```python
from build123d import *

# Parameters (mm, degrees)
SKETCH1_W                = 90
SKETCH1_H                = 29
SKETCH1_W_2              = 86
SKETCH1_H_2              = 25
BOSS_EXTRUDE1_DEPTH      = 12
SKETCH1_2_W              = 90
SKETCH1_2_H              = 29
SKETCH1_2_W_2            = 86
SKETCH1_2_H_2            = 25
BOSS_EXTRUDE2_DEPTH      = 2
SKETCH2_R                = 1
BOSS_EXTRUDE3_DEPTH      = 2.65
SKETCH3_R                = 1.75
BOSS_EXTRUDE4_DEPTH      = 1
CHAMFER1_SIZE            = 1
CUT_EXTRUDE1_REACH       = 55.833
SKETCH4_W                = 13
SKETCH4_H                = 10
CUT_EXTRUDE2_REACH       = 56.863
SKETCH5_W                = 24
SKETCH5_H                = 3
CHAMFER2_SIZE            = 1
CHAMFER2_OF_MIRROR2_SIZE = 1


with BuildPart() as part:
    # Sketch1 → Boss-Extrude1 (new body)
    with BuildSketch(Plane(origin=(0, 0, 0), x_dir=(1, 0, 0), z_dir=(0, 1, 0))):
        Rectangle(SKETCH1_W, SKETCH1_H)
        Rectangle(SKETCH1_W_2, SKETCH1_H_2, mode=Mode.SUBTRACT)
    extrude(amount=BOSS_EXTRUDE1_DEPTH)

    # Sketch1_2 → Boss-Extrude2 (add)
    # profile 1 of 2: a face of its own
    with BuildSketch(Plane(origin=(0, 0, 0), x_dir=(1, 0, 0), z_dir=(0, 1, 0))):
        Rectangle(SKETCH1_2_W, SKETCH1_2_H)
        Rectangle(SKETCH1_2_W_2, SKETCH1_2_H_2, mode=Mode.SUBTRACT)
    # profile 2 of 2: a face of its own
    with BuildSketch(Plane(origin=(0, 0, 0), x_dir=(1, 0, 0), z_dir=(0, 1, 0))):
        Rectangle(SKETCH1_2_W_2, SKETCH1_2_H_2)
    extrude(amount=-BOSS_EXTRUDE2_DEPTH)

    # Sketch2 → Boss-Extrude3 (add)
    with BuildSketch(Plane(origin=(0, 0, 0), x_dir=(1, 0, 0), z_dir=(0, 1, 0))):
        with Locations(Location((40.6, -10.1, 0), (0, 0, 270))):
            Circle(SKETCH2_R)
        with Locations(Location((-40.6, -10.1, 0), (0, 0, 90))):
            Circle(SKETCH2_R)
    extrude(amount=BOSS_EXTRUDE3_DEPTH)

    # Sketch3 → Boss-Extrude4 (add)
    with BuildSketch(Plane(origin=(0, 0, 0), x_dir=(1, 0, 0), z_dir=(0, 1, 0))):
        with Locations(Location((40.6, -10.1, 0), (0, 0, 270))):
            Circle(SKETCH3_R)
        with Locations(Location((-40.6, -10.1, 0), (0, 0, 270))):
            Circle(SKETCH3_R)
    boss_extrude4 = extrude(amount=BOSS_EXTRUDE4_DEPTH)

    # Mirror1: Boss-Extrude4 across plane
    add(boss_extrude4.mirror(Plane.XY))

    # Chamfer1
    chamfer1_edges = [part.edges().sort_by_distance(p)[0] for p in [
        (0, -2, 14.5),
        (45, -2, 0),
        (-45, -2, 0),
        (0, -2, -14.5),
        (45, 5, 14.5),
        (-45, 5, 14.5),
        (-45, 5, -14.5),
        (45, 5, -14.5),
    ]]
    chamfer(chamfer1_edges, length=CHAMFER1_SIZE)

    # Sketch4 → Cut-Extrude1 (cut, up to next)
    with BuildSketch(Plane(origin=(0, 0, -12.5), x_dir=(-1, 0, 0), z_dir=(0, 0, -1)), mode=Mode.PRIVATE) as cut_extrude1_sk1:
        with Locations((0, 7)):
            Rectangle(SKETCH4_W, SKETCH4_H)
    cut_extrude1_tool1 = extrude(cut_extrude1_sk1.sketch, amount=CUT_EXTRUDE1_REACH, mode=Mode.PRIVATE) & part.part
    add(cut_extrude1_tool1.solids().sort_by_distance((0, 7, -12.5))[0], mode=Mode.SUBTRACT)

    # Sketch5 → Cut-Extrude2 (cut, up to next)
    with BuildSketch(Plane(origin=(0, 0, -14.5), x_dir=(-1, 0, 0), z_dir=(0, 0, -1)), mode=Mode.PRIVATE) as cut_extrude2_sk1:
        with Locations((-24, 3.5)):
            Rectangle(SKETCH5_W, SKETCH5_H)
    cut_extrude2_tool1 = extrude(cut_extrude2_sk1.sketch, amount=-CUT_EXTRUDE2_REACH, mode=Mode.PRIVATE) & part.part
    cut_extrude2 = cut_extrude2_tool1.solids().sort_by_distance((24, 3.5, -14.5))[0]
    add(cut_extrude2, mode=Mode.SUBTRACT)

    # Chamfer2
    chamfer2_edges = [part.edges().sort_by_distance(p)[0] for p in [
        (12, 3.5, -14.5),
        (24, 5, -14.5),
        (36, 3.5, -14.5),
        (24, 2, -14.5),
    ]]
    chamfer(chamfer2_edges, length=CHAMFER2_SIZE)

    # Mirror2: Cut-Extrude2 across plane
    add(cut_extrude2.mirror(Plane(origin=(0, 0, 0), x_dir=(0, 0, 1), z_dir=(1, 0, 0))), mode=Mode.SUBTRACT)

    # Chamfer2 of Mirror2
    chamfer2_of_mirror2_edges = [part.edges().sort_by_distance(p)[0] for p in [
        (-12, 3.5, -14.5),
        (-24, 5, -14.5),
        (-36, 3.5, -14.5),
        (-24, 2, -14.5),
    ]]
    chamfer(chamfer2_of_mirror2_edges, length=CHAMFER2_OF_MIRROR2_SIZE)


solid = part.part
```
The listing builds one solid part. Answer for the finished solid, in the listing's coordinates (mm). A direction names the side the tool comes from. Coordinates: 2 decimals unless noted, no trailing zeros. Write each loop counter-clockwise with the first axis right and the second up, starting at its lowest first coordinate (ties: lowest second). Pieces come first, ordered by that corner, then holes. Notation, with made-up numbers: (40.25, 75.25) - (69.25, 75.25) arc R18 cw to (69.25, 99.25) - close; hole circle Ø9 at (23.5, 44.5). An arc over 180 degrees is marked (long way). One line per item, written item: value.
1) Find section A-A (x = -17.5). Give the vertices of the cut face in (y, z), and give its area (3 significant figures).
Geometry check:
outline: (-2, -13.5) - (-1, -14.5) - (1, -14.5) - (2, -13.5) - (2, -12.5) - (0, -12.5) - (0, 12.5) - (12, 12.5) - (12, 14.5) - (-1, 14.5) - (-2, 13.5) - close; (5, -13.5) - (6, -14.5) - (12, -14.5) - (12, -12.5) - (5, -12.5) - close
area: 98.0 mm2
2) Find section B-B (z = 2). Give the vertices of the cut face in (x, y), and give its area (3 significant figures).
Geometry check:
outline: (-45, -1) - (-44, -2) - (44, -2) - (45, -1) - (45, 12) - (43, 12) - (43, 0) - (-43, 0) - (-43, 12) - (-45, 12) - close
area: 227 mm2
3) Find section C-C (x = 40.6). Give the vertices of the cut face in (y, z), and give its area (3 significant figures).
Geometry check:
outline: (-2, -13.5) - (-1, -14.5) - (12, -14.5) - (12, -12.5) - (0, -12.5) - (0, -11.85) - (1, -11.85) - (1, -8.35) - (0, -8.35) - (0, 8.35) - (1, 8.35) - (1, 9.1) - (2.65, 9.1) - (2.65, 11.1) - (1, 11.1) - (1, 11.85) - (0, 11.85) - (0, 12.5) - (12, 12.5) - (12, 14.5) - (-1, 14.5) - (-2, 13.5) - close
area: 115 mm2
4) For a pull along X with two mould halves and no side action, classify faces 1 (the flat face through (-1, -2, 0)), 2 (the flat face through (45, 6, 0)), 3 (the flat face through (-6.5, 7, -13)) as pulls with the +X half, pulls with the -X half, needs draft (parallel to the pull), parting line crosses it, or undercut.
Geometry check:
face 1: needs draft
face 2: pulls with the +X half
face 3: undercut
5) Find section D-D (z = 10.1). Give the vertices of the cut face in (x, y).
Geometry check:
outline: (-45, -1) - (-44, -2) - (44, -2) - (45, -1) - (45, 12) - (43, 12) - (43, 0) - (42.35, 0) - (42.35, 1) - (41.6, 1) - (41.6, 2.65) - (39.6, 2.65) - (39.6, 1) - (38.85, 1) - (38.85, 0) - (-38.85, 0) - (-38.85, 1) - (-39.6, 1) - (-39.6, 2.65) - (-41.6, 2.65) - (-41.6, 1) - (-42.35, 1) - (-42.35, 0) - (-43, 0) - (-43, 12) - (-45, 12) - close
6) Consider line 1 along Z through (x, y) = (-19, 10.75); line 2 along X through (y, z) = (8.25, 5); line 3 along Y through (x, z) = (23, 5.5). Determine where each line is inside the solid, lowest interval first. Write a range as from..to.
Geometry check:
line 1: z = -14.5..-12.5, 12.5..14.5
line 2: x = -45..-43, 43..45
line 3: y = -2..0
7) A tool of negligible diameter and unlimited length cuts with its end or side. For faces 4 (the flat face through (0, 12, 13)), 5 (the flat face through (0, 2, -13)), 6 (the cylindrical face through (-40.074, 0.493, 11.769)), from which of +Z, -Z, +X, -X, +Y, -Y can it reach the whole face along a straight path? Write none if from no direction.
Geometry check:
face 4: +Z, -Z, +X, -X, +Y
face 5: -Z, +Y
face 6: +Y
8) Each of these flat-tipped pins is pushed along its axis until it touches: pin 1 Ø8 at (x, z) = (4.5, 1.5) entering from +Y; pin 2 Ø4 at (x, z) = (40.5, 10) entering from +Y; pin 3 Ø1.6 at (x, z) = (-2.5, -13.5) entering from +Y. Where does it stop, or does it pass through?
Geometry check:
pin 1: stops at y = 0
pin 2: stops at y = 2.65
pin 3: stops at y = 2
